from build123d import *

# Parameters (mm, degrees)
F1_DEPTH = 9.525


with BuildPart() as f1:
    # F0 (on Top) → F1 (new body)
    with BuildSketch(Plane.XY):
        with BuildLine():
            Line((-77.7875, -66.675), (77.7875, -66.675))
            ThreePointArc((77.7875, -66.675), (87.890288, -62.490288), (92.075, -52.3875))
            Line((92.075, -52.3875), (92.075, 52.3875))
            ThreePointArc((92.075, 52.3875), (87.890288, 62.490288), (77.7875, 66.675))
            Line((77.7875, 66.675), (-77.7875, 66.675))
            ThreePointArc((-77.7875, 66.675), (-87.890288, 62.490288), (-92.075, 52.3875))
            Line((-92.075, 52.3875), (-92.075, -52.3875))
            ThreePointArc((-92.075, -52.3875), (-87.890288, -62.490288), (-77.7875, -66.675))
        make_face()
        with BuildLine():
            ThreePointArc((-74.240388, -57.654424), (-83.054424, -55.934612), (-81.334612, -47.120576))
            Line((-81.334612, -47.120576), (-70.222112, -39.636647))
            ThreePointArc((-70.222112, -39.636647), (-61.408076, -41.356459), (-63.127888, -50.170496))
            Line((-63.127888, -50.170496), (-74.240388, -57.654424))
        make_face(mode=Mode.SUBTRACT)
        with BuildLine():
            ThreePointArc((81.334612, -47.120576), (83.054424, -55.934612), (74.240388, -57.654424))
            Line((74.240388, -57.654424), (63.127888, -50.170496))
            ThreePointArc((63.127888, -50.170496), (61.408076, -41.356459), (70.222112, -39.636647))
            Line((70.222112, -39.636647), (81.334612, -47.120576))
        make_face(mode=Mode.SUBTRACT)
        with BuildLine():
            ThreePointArc((-81.334612, 47.120576), (-83.054424, 55.934612), (-74.240388, 57.654424))
            Line((-74.240388, 57.654424), (-63.127888, 50.170496))
            ThreePointArc((-63.127888, 50.170496), (-61.408076, 41.356459), (-70.222112, 39.636647))
            Line((-70.222112, 39.636647), (-81.334612, 47.120576))
        make_face(mode=Mode.SUBTRACT)
        with BuildLine():
            ThreePointArc((74.240388, 57.654424), (83.054424, 55.934612), (81.334612, 47.120576))
            Line((81.334612, 47.120576), (70.222112, 39.636647))
            ThreePointArc((70.222112, 39.636647), (61.408076, 41.356459), (63.127888, 50.170496))
            Line((63.127888, 50.170496), (74.240388, 57.654424))
        make_face(mode=Mode.SUBTRACT)
    extrude(amount=-F1_DEPTH)


solid = f1.part
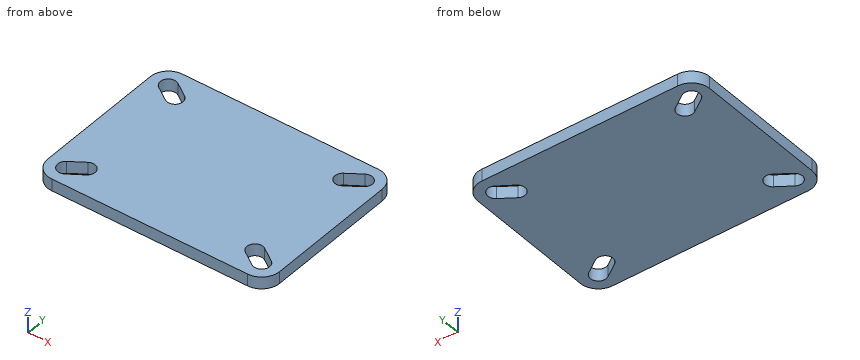
The listing builds one solid part. Answer for the finished solid, in the listing's coordinates (mm). Round coordinates to 2 decimals unless told otherwise and drop trailing zeros. Write each loop counter-clockwise with the first axis right and the second up, starting at its lowest first coordinate (ties: lowest second). Pieces come first, ordered by that corner, then holes. Notation, with made-up numbers: (59.5, 42.25) - (96.5, 42.25) arc R20 ccw to (96.5, 73.25) - close; hole circle Ø11 at (11.5, 20). An arc over 180 degrees is marked (long way). Use one line per item in the form item = value. Start each with the question number.
Item 1: A cutting plane is placed at B-B (y = -43.5). Write down the section's boundary in (x, z) (3 decimals), plus the area to 3 significant figures.
Item 2: Find the intervals of material crossed by line 1 (Y direction, x = -78, z = -5); line 2 (X direction, y = 53, z = -2); line 3 (X direction, y = 45, z = -7) (3 decimals), in increasing order. Write a range as [from, to].
Item 3: A cutting plane is placed at A-A (z = -6.5). Give the number of separate pieces and of enclosed holes in the cut face, plus the area to 3 significant figures.
Item 4: A cutting plane is placed at C-C (x = 67.5). Write down the section's boundary in (y, z) (3 decimals).
The answers:
q1.outline = (-92.075, -9.525) - (-75.959, -9.525) - (-75.959, 0) - (-92.075, 0) - close; (-60.482, -9.525) - (60.482, -9.525) - (60.482, 0) - (-60.482, 0) - close; (75.959, -9.525) - (92.075, -9.525) - (92.075, 0) - (75.959, 0) - close
q1.area = 1,460 mm^2
q2.line_1 = [-66.67, -58.73], [-44.87, 44.87], [58.73, 66.67]
q2.line_2 = [-92.06, -84.11], [-67.33, 67.33], [84.11, 92.06]
q2.line_3 = [-92.075, -78.186], [-60.326, 60.326], [78.186, 92.075]
q3.separate_pieces = 1
q3.enclosed_holes = 4
q3.area = 23,200 mm^2
q4.outline = (-66.675, -9.525) - (-53.115, -9.525) - (-53.115, 0) - (-66.675, 0) - close; (-38.607, -9.525) - (38.607, -9.525) - (38.607, 0) - (-38.607, 0) - close; (53.115, -9.525) - (66.675, -9.525) - (66.675, 0) - (53.115, 0) - close
